Input: part model. Units: mm. Frame: model coordinates. Coordinates: 2 decimals unless noted, no trailing zeros. Loops run counter-clockwise (first coordinate to the right, second up) from the corner with the lowest first, then second, coordinate; pieces in that order, holes last.
```python
from build123d import *

# Parameters (mm, degrees)
SKETCH4_W           = 28
SKETCH4_H           = 45
BOSS_EXTRUDE2_DEPTH = 10
SKETCH6_R           = 1.7
CUT_EXTRUDE1_DEPTH  = 29.324018077


with BuildPart() as part:
    # Sketch4 → Boss-Extrude2 (new body)
    with BuildSketch(Plane.XY):
        Rectangle(SKETCH4_W, SKETCH4_H)
    extrude(amount=BOSS_EXTRUDE2_DEPTH)

    # Sketch5 → Cut-Revolve1 (revolve, cut)
    with BuildSketch(Plane.XY):
        Polygon((0, 22.5), (8.33, 22.5), (8.33, 16.5), (6, 10.5), (4.75, -18.71), (4.75, -22.5), (0, -22.5), align=None)
    revolve(axis=Axis((0, 0, 0), (0, 1, 0)), mode=Mode.SUBTRACT)

    # Sketch6 → Cut-Extrude1 (cut, through all)
    with BuildSketch(Plane.XY.offset(10)):
        with Locations((-10.5, 6.5)):
            Circle(SKETCH6_R)
        with Locations((-10.5, -17.5)):
            Circle(SKETCH6_R)
        with Locations((10.5, 6.5)):
            Circle(SKETCH6_R)
        with Locations((10.5, -17.5)):
            Circle(SKETCH6_R)
    extrude(amount=-CUT_EXTRUDE1_DEPTH, mode=Mode.SUBTRACT)


solid = part.part
```
Item 1: Section query A-A (x = -10.5). Output: boundary loops of the cut face in (y, z).
Result:
outline: (-22.5, 0) - (-19.2, 0) - (-19.2, 10) - (-22.5, 10) - close; (-15.8, 0) - (4.8, 0) - (4.8, 10) - (-15.8, 10) - close; (8.2, 0) - (22.5, 0) - (22.5, 10) - (8.2, 10) - close
Item 2: Mould query, pull axis Y, two halves, no side actions, for faces 1 (the face through (-0.18, 19.46, 8.33)), 2 (the face through (-0.152, 12.791, 6.888)), 3 (the face through (12.12, -16.99, 5.07)). Classes: +Y half, -Y half, draft (parallel to the pull), parting line (faces both ways), or undercut.
Result:
face 1: draft
face 2: +Y half
face 3: undercut
Item 3: Line query: L1, parallel to Y at x = 10.5, z = 7; L2, parallel to Y at x = 9.75, z = 7.25; L3, parallel to X at y = 5, z = 5.25. Output: solid intervals per line, ascending.
Result:
L1: y = -22.5 to -19.2, -15.8 to 4.8, 8.2 to 22.5
L2: y = -22.5 to -19.03, -15.97 to 4.97, 8.03 to 22.5
L3: x = -14 to -11.3, -9.7 to -2.38, 2.38 to 9.7, 11.3 to 14
Item 4: Section query D-D (z = 2.25). Count the separate pieces of the cut face and the enclosed holes in it, then the cut area to 3 significant figures.
Result:
separate pieces: 2
enclosed holes: 4
area: 729 mm2
Item 5: Section query B-B (y = -17.5). Output: boundary loops of the cut face in (x, z).
Result:
outline: (-14, 0) - (-12.2, 0) - (-12.2, 10) - (-14, 10) - close; (-8.8, 0) - (-4.8, 0) arc R4.8 cw to (4.8, 0) - (8.8, 0) - (8.8, 10) - (-8.8, 10) - close; (12.2, 0) - (14, 0) - (14, 10) - (12.2, 10) - close
Item 6: Section query C-C (x = 0). Output: boundary loops of the cut face in (y, z), then the cut area to 3 significant figures.
Result:
outline: (-22.5, 4.75) - (-18.71, 4.75) - (10.5, 6) - (16.5, 8.33) - (22.5, 8.33) - (22.5, 10) - (-22.5, 10) - close
area: 182 mm2
Item 7: Contact query for flat-ended pins moving along their axis: P1, Ø2, axis at x = -3.5, y = 10.5, coming from the -Z side; P2, Ø4, axis at x = 0.5, y = 6.5, coming from the -Z side. Output: stop coordinate, or through.
Result:
P1: stops at z = 3.97
P2: stops at z = 5.26
